Work out the finished part from the listing and answer in its coordinate system (mm). A direction names the side the tool comes from. Round coordinates to 2 decimals unless told otherwise and drop trailing zeros. Write each loop counter-clockwise with the first axis right and the second up, starting at its lowest first coordinate (ties: lowest second). Pieces come first, ordered by that corner, then holes.
from build123d import *

# Parameters (mm, degrees)
SKETCH1_R          = 2
BASE_EXTRUDE_DEPTH = 65.085
SKETCH2_R          = 5
PISTON_DEPTH       = 2.5


with BuildPart() as part:
    # Sketch1 → Base-Extrude (new body)
    with BuildSketch(Plane.XY):
        Circle(SKETCH1_R)
    extrude(amount=BASE_EXTRUDE_DEPTH)

    # Sketch2 → Piston (add, symmetric)
    with BuildSketch(Plane.XY):
        Circle(SKETCH2_R)
    extrude(amount=PISTON_DEPTH, both=True)

    # Sketch3 → Threads (revolve, cut)
    with BuildSketch(Plane(origin=(0, 0, 0), x_dir=(0, 0, -1), z_dir=(1, 0, 0))):
        Polygon((-65.085, 1.5525), (-64.885, 1.7525), (-50.085, 1.7525), (-50.085, 1.55), (-48.885, 1.55), (-48.685, 1.75), (-48.685, 5), (-65.085, 5), align=None)
    revolve(axis=Axis((0, 0, 0), (0, 0, 1)), mode=Mode.SUBTRACT)


solid = part.part
Q1. Find section D-D (y = -3). Determine the outline of the cut face in (x, z).
Q2. Given pin 1 (3 mm diameter, centred on x = 2.5, z = 52, fed in from -Y); pin 2 (4 mm diameter, centred on x = -0.5, z = 40.5, fed in from -Y); pin 3 (4 mm diameter, centred on y = 0.5, z = 28, fed in from -X); pin 4 (1 mm diameter, centred on x = -3, z = 55.5, fed in from -Y), each flat-ended and moving along its own axis, determine where each tip first touches the part or whether it passes through.
Q3. The mould has two halves that part along Z. Classify faces 1 (the face through (-1.08, -4.88, 0.04)), 2 (the face through (0, 0, -2.5)), 3 (the face through (-0.1, -2.2, 2.5)), 4 (the face through (1.375, 0.715, 49.477)): +Z half, -Z half, draft (parallel to the pull), parting line (faces both ways), or undercut.
Q4. Find section C-C (z = 17.5). Determine the outline of the cut face in (x, y), plus the area to 3 significant figures.
Q5. A tool of negligible diameter and unlimited length cuts with its end or side. For faces 5 (the face through (0, -2, 25)), 6 (the face through (0, 0, 65.085)), from which of +Z, -Z, +X, -X, +Y, -Y can it reach the whole face along a straight path? Write none if from no direction.
Q6. Find the intervals of material crossed by L1, parallel to X at y = 0, z = 43.5; L2, parallel to Z at x = -2.25, y = -2.5; L3, parallel to Y at x = 1.25, z = 18, in increasing order.
Report:
1. outline: (-4, -2.5) - (4, -2.5) - (4, 2.5) - (-4, 2.5) - close
2. pin 1: stops at y = -1.44
2. pin 2: stops at y = -2
2. pin 3: stops at x = -2
2. pin 4: passes through
3. face 1: draft
3. face 2: -Z half
3. face 3: +Z half
3. face 4: undercut
4. outline: circle Ø4 at (0, 0)
4. area: 12.6 mm2
5. face 5: +Z
5. face 6: +Z, +X, -X, +Y, -Y
6. L1: x = -2 to 2
6. L2: z = -2.5 to 2.5
6. L3: y = -1.56 to 1.56
